from build123d import *

# Parameters (mm, degrees)
SKETCH1_R           = 7.75
SKETCH1_R_2         = 5.25
BOSS_EXTRUDE1_DEPTH = 1
SKETCH2_R           = 6.75
SKETCH2_R_2         = 5.25
BOSS_EXTRUDE2_DEPTH = 3.5
CHAMFER1_SIZE       = 1


with BuildPart() as part:
    # Sketch1 → Boss-Extrude1 (new body)
    with BuildSketch(Plane.XY):
        Circle(SKETCH1_R)
        Circle(SKETCH1_R_2, mode=Mode.SUBTRACT)
    extrude(amount=BOSS_EXTRUDE1_DEPTH)

    # Sketch2 → Boss-Extrude2 (add)
    with BuildSketch(Plane.XY.offset(1)):
        Circle(SKETCH2_R)
        Circle(SKETCH2_R_2, mode=Mode.SUBTRACT)
    extrude(amount=BOSS_EXTRUDE2_DEPTH)

    # Chamfer1
    chamfer1_edges = [part.edges().sort_by_distance(p)[0] for p in [
        (-6.75, 0, 1),
    ]]
    chamfer(chamfer1_edges, length=CHAMFER1_SIZE - 0.0001)  # a hair under: the kernel refuses the full size

    # Mirror5: part across plane


with BuildPart() as part_1:
    add(part.part)
    add(part.part.mirror(Plane.XY.offset(4.5)))


solid = part_1.part
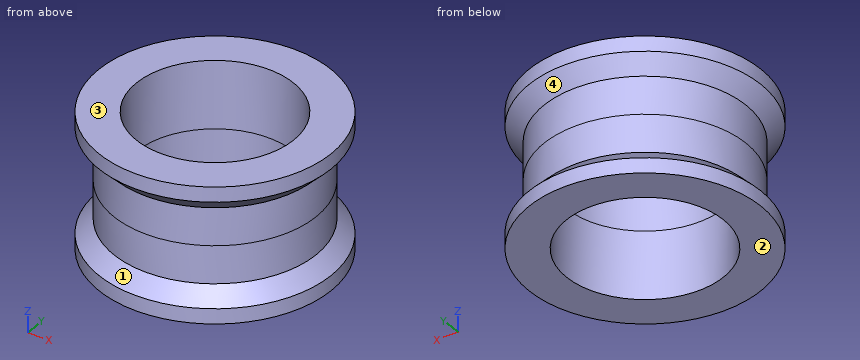
The model under review builds one solid part; all positions refer to its coordinate system, in mm. Face numbers are marked on the shaded views. Give positions to 0.01 mm unless a question says otherwise; leave off trailing zeros. Loops run counter-clockwise (first coordinate to the right, second up) from the corner with the lowest first, then second, coordinate; pieces in that order, holes last. Notation, with made-up numbers: (-0.5, 36) -> (24.5, 36) arc R9 cw to (24.5, 40) -> close; hole circle Ø9 at (-5, 47). An arc over 180 degrees is marked (long way). Answer as a JSON object with one key per item and string values. Group by question number.
Q1. Take a section at C-C (z = 0.5). Write out the cut boundary in (x, y).
Q2. Wall thickness on line 1 along Y through (x, z) = (0, 3.4); line 2 along Z through (x, y) = (-6.75, -2.25); line 3 along Y through (x, z) = (4.25, 1.5): over which ranges is each line inside the solid? List them lowest first.
Q3. Draft analysis for pull direction Z (two halves, no side actions). For the marked faces 1, 2, 3 and 4, state which applies: pulls with the +Z half, pulls with the -Z half, needs draft (parallel to the pull), parting line crosses it, or undercut.
Q4. Take a section at D-D (z = 6.5). Write out the cut boundary in (x, y), plus the area to 3 significant figures.
Q5. Insertion check: pin 1 (5 mm diameter, centred on x = 3, z = 6.5, fed in from +Y); pin 2 (5 mm diameter, centred on y = 4.5, z = 5, fed in from +X). Each pin has a flat end and moves straight along its axis. Give the tip position at first contact, or say it passes through.
Answer below:
{
 "1": {"outline": "circle Ø15.5 at (0, 0); hole circle Ø10.5 at (0, 0)"},
 "2": {"line 1": "y = -6.75 to -5.25, 5.25 to 6.75", "line 2": "z = 0 to 1.63, 7.37 to 9", "line 3": "y = -5.87 to -3.08, 3.08 to 5.87"},
 "3": {"face 1": "undercut", "face 2": "pulls with the -Z half", "face 3": "pulls with the +Z half", "face 4": "undercut"},
 "4": {"outline": "circle Ø13.5 at (0, 0); hole circle Ø10.5 at (0, 0)", "area": "56.5 mm2"},
 "5": {"pin 1": "stops at y = 7.69", "pin 2": "stops at x = 6.45"}
}
